Verification items for the finished model (mm, model axes). A direction names the side the tool comes from. Give positions to 0.01 mm unless a question says otherwise; leave off trailing zeros. Write each loop counter-clockwise with the first axis right and the second up, starting at its lowest first coordinate (ties: lowest second). Pieces come first, ordered by that corner, then holes. Notation, with made-up numbers: M 80.5,51 L 107.5,51 A31 ccw 107.5,76 Z; hole C 8,-23.75 d3. An arc over 180 degrees is marked long. Write item = value, one per line.
from build123d import *

# Parameters (mm, degrees)
SKETCH3_R               = 1.7
CUT_EXTRUDE1_DEPTH      = 68.372101051
CIRPATTERN1_COUNT       = 4
BOSS_EXTRUDE1_DEPTH     = 11
SKETCH6_R               = 8.4
CUT_EXTRUDE2_DEPTH      = 3
SKETCH7_W               = 6.9
SKETCH7_H               = 40
CUT_EXTRUDE3_DEPTH      = 4
SKETCH8_R               = 1.7
CUT_EXTRUDE4_DEPTH      = 68.727394753
SKETCH9_R               = 4
BOSS_EXTRUDE2_DEPTH     = 6.5
SKETCH10_R              = 1.7
CUT_EXTRUDE5_DEPTH      = 69.733179761
CUT_EXTRUDE6_DEPTH      = 1
CUT_EXTRUDE6_DEPTH_BACK = 3
SKETCH12_R              = 2.95
CUT_EXTRUDE7_DEPTH      = 3
CIRPATTERN2_COUNT       = 4
CUT_EXTRUDE8_DEPTH      = 3


with BuildPart() as part:
    # Sketch1 → Revolve1 (revolve)
    with BuildSketch(Plane.XY):
        Polygon((25, 0), (47, 0), (47, -5), (35, -5), (35, -11), (25, -11), align=None)
    revolve(axis=Axis((0, -62.255842479, 0), (0, 1, 0)))

    # Sketch3 → Cut-Extrude1 (cut, symmetric)
    with BuildSketch(Plane(origin=(0, 0, 0), x_dir=(1, 0, 0), z_dir=(0, 1, 0))):
        with Locations(Location((21.213203436, 21.213203436, 0), (0, 0, 180))):
            Circle(SKETCH3_R)
    cut_extrude1 = extrude(amount=CUT_EXTRUDE1_DEPTH, both=True, mode=Mode.SUBTRACT)

    # CirPattern1: Cut-Extrude1 ×4 about axis
    cirpattern1_axis = Axis((0, 0, 0), (0, 1, 0))
    for i in range(1, CIRPATTERN1_COUNT):
        add(cut_extrude1.rotate(cirpattern1_axis, i * 360 / CIRPATTERN1_COUNT), mode=Mode.SUBTRACT)

    # Sketch4 → Boss-Extrude1 (add, through all)
    with BuildSketch(Plane(origin=(0, 0, 0), x_dir=(1, 0, 0), z_dir=(0, 1, 0))):
        with BuildLine():
            ThreePointArc((4.118263467, 16.493632287), (-12.020815273, 12.020815288), (-16.493632292, -4.118263447))
            ThreePointArc((-16.493632292, -4.118263447), (-19.405482869, -8.968121999), (-24.255341261, -6.056271155))
            ThreePointArc((-24.255341261, -6.056271155), (17.677669687, -17.677669372), (6.056270723, 24.255341369))
            ThreePointArc((6.056270723, 24.255341369), (8.968122055, 19.405483096), (4.118263467, 16.493632287))
        make_face()
    extrude(amount=-BOSS_EXTRUDE1_DEPTH)

    # Sketch5 → Revolve2 (revolve)
    with BuildSketch(Plane(origin=(0, 0, 0), x_dir=(0, 0, -1), z_dir=(1, 0, 0)), mode=Mode.PRIVATE) as revolve2_sk:
        Polygon((-8.4, 0), (-8.4, 6), (-11.8, 6), (-17, 0), align=None)
    revolve(revolve2_sk.sketch.rotate(Axis((0, 0, 0), (0, -1, 0)), 194.019424572), axis=Axis((0, 0, 0), (0, -1, 0)))

    # Sketch6 → Cut-Extrude2 (cut)
    with BuildSketch(Plane(origin=(0, 0, 0), x_dir=(1, 0, 0), z_dir=(0, 1, 0))):
        with Locations(Location((0, 0, 0), (0, 0, 270))):
            Circle(SKETCH6_R)
    extrude(amount=-CUT_EXTRUDE2_DEPTH, mode=Mode.SUBTRACT)

    # Sketch7 → Cut-Extrude3 (cut)
    with BuildSketch(Plane(origin=(0, 6, 0), x_dir=(1, 0, 0), z_dir=(0, 1, 0))):
        Rectangle(SKETCH7_W, SKETCH7_H)
    extrude(amount=-CUT_EXTRUDE3_DEPTH, mode=Mode.SUBTRACT)

    # Sketch8 → Cut-Extrude4 (cut, through all)
    with BuildSketch(Plane(origin=(0, 2, 0), x_dir=(1, 0, 0), z_dir=(0, 1, 0))):
        with Locations(Location((0, 11, 0), (0, 0, 270))):
            Circle(SKETCH8_R)
        with Locations(Location((0, -11, 0), (0, 0, 270))):
            Circle(SKETCH8_R)
    extrude(amount=-CUT_EXTRUDE4_DEPTH, mode=Mode.SUBTRACT)

    # Sketch9 → Boss-Extrude2 (add)
    with BuildSketch(Plane(origin=(0, 0, 0), x_dir=(1, 0, 0), z_dir=(0, 1, 0))):
        with Locations((43, 0)):
            Circle(SKETCH9_R)
        with Locations(Location((15, 0, 0), (0, 0, 293.578178493))):
            Circle(SKETCH9_R)
    extrude(amount=BOSS_EXTRUDE2_DEPTH)

    # Sketch10 → Cut-Extrude5 (cut, through all)
    with BuildSketch(Plane(origin=(0, 6.5, 0), x_dir=(1, 0, 0), z_dir=(0, 1, 0))):
        with Locations(Location((15, 0, 0), (0, 0, 180))):
            Circle(SKETCH10_R)
        with Locations(Location((43, 0, 0), (0, 0, 180))):
            Circle(SKETCH10_R)
    extrude(amount=-CUT_EXTRUDE5_DEPTH, mode=Mode.SUBTRACT)

    # Sketch11 → Cut-Extrude6 (cut, two sides: drawn at the far end of the back side and taken through both)
    with BuildSketch(Plane(origin=(0, 3.5, 0), x_dir=(1, 0, 0), z_dir=(0, 1, 0)).offset(-CUT_EXTRUDE6_DEPTH_BACK)):
        Polygon((18.35, 0), (16.675, 2.901185103), (13.325, 2.901185103), (11.65, 0), (13.325, -2.901185103), (16.675, -2.901185103), align=None)
        Polygon((41.325, 2.901185103), (44.675, 2.901185103), (46.35, 0), (44.675, -2.901185103), (41.325, -2.901185103), (39.65, 0), align=None)
        Polygon((16.675, -2.901185103), (18.35, 0), (16.675, 2.901185103), (41.325, 2.901185103), (39.65, 0), (41.325, -2.901185103), align=None)
    extrude(amount=CUT_EXTRUDE6_DEPTH + CUT_EXTRUDE6_DEPTH_BACK, mode=Mode.SUBTRACT)

    # Sketch12 → Cut-Extrude7 (cut)
    with BuildSketch(Plane(origin=(0, 0, 0), x_dir=(1, 0, 0), z_dir=(0, 1, 0))):
        with Locations(Location((-21.213203436, 21.213203436, 0), (0, 0, 180))):
            Circle(SKETCH12_R)
    cut_extrude7 = extrude(amount=-CUT_EXTRUDE7_DEPTH, mode=Mode.SUBTRACT)

    # CirPattern2: Cut-Extrude7 ×4 about axis
    cirpattern2_axis = Axis((0, 0, 0), (0, 1, 0))
    for i in range(1, CIRPATTERN2_COUNT):
        add(cut_extrude7.rotate(cirpattern2_axis, i * 360 / CIRPATTERN2_COUNT), mode=Mode.SUBTRACT)

    # Sketch14 → Cut-Extrude8 (cut)
    with BuildSketch(Plane.XZ.offset(11)):
        Polygon((-1.675, 13.901185103), (1.675, 13.901185103), (3.35, 11), (1.675, 8.098814897), (-1.675, 8.098814897), (-3.35, 11), align=None)
        Polygon((-1.675, -8.098814897), (-3.35, -11), (-1.675, -13.901185103), (1.675, -13.901185103), (3.35, -11), (1.675, -8.098814897), align=None)
    extrude(amount=-CUT_EXTRUDE8_DEPTH, mode=Mode.SUBTRACT)


solid = part.part
1) Cross-section at A-A on x = 43. Record the boundary of the cut face in (y, z), plus the area to 3 significant figures.
From the geometry:
outline = M -5,-18.97 L 0,-18.97 L 0,-4 L 6.5,-4 L 6.5,-1.7 L 4.5,-1.7 L 4.5,-2.9 L 0.5,-2.9 L 0.5,-1.7 L -5,-1.7 Z; M -5,1.7 L 0.5,1.7 L 0.5,2.9 L 4.5,2.9 L 4.5,1.7 L 6.5,1.7 L 6.5,4 L 0,4 L 0,18.97 L -5,18.97 Z
area = 193 mm^2
2) Depth check by flat-ended pin: P1, Ø7, axis at x = -21.21, z = -21.21, coming from the +Y side; P2, Ø3.5, axis at x = -21.21, z = 21.21, coming from the +Y side; P3, Ø8, axis at y = 1.5, z = -8.5, coming from the +X side; P4, Ø6, axis at x = -2, z = -21.5, coming from the -Y side. Enter the tip coordinate at first touch or a pass-through.
From the geometry:
P1 = 0
P2 = -3
P3 = 46.76
P4 = through
3) Cross-section at B-B on z = -31. Record the boundary of the cut face in (x, y).
From the geometry:
outline = M -35.33,-5 L -16.25,-5 L -16.25,-11 L 16.25,-11 L 16.25,-5 L 35.33,-5 L 35.33,0 L -35.33,0 Z
4) Cross-section at C-C on x = 26.5. Record the boundary of the cut face in (y, z), plus the area to 3 significant figures.
From the geometry:
outline = M -11,-22.86 L -5,-22.86 L -5,-38.82 L 0,-38.82 L 0,38.82 L -5,38.82 L -5,22.86 L -11,22.86 Z
area = 663 mm^2
5) Cross-section at D-D on z = 38.5. Record the boundary of the cut face in (x, y).
From the geometry:
outline = M -26.96,-5 L 26.96,-5 L 26.96,0 L -26.96,0 Z
6) Draft check along Y on faces 1 (the flat face through (17, 4.5, 0)), 2 (the flat face through (-2.5, -9.52, 9.53)), 3 (the flat face through (-1.4, -8, 12.3)). Enter one of: +Y half, -Y half, draft (parallel to the pull), parting line (faces both ways), or undercut.
From the geometry:
face_1 = undercut
face_2 = draft
face_3 = -Y half
7) Material ranges on probe 1 along X at (y, z) = (-4, -10); probe 2 along X at (y, z) = (-2.5, -11); probe 3 along Z at (x, y) = (-7, -2), recorded low to high. Write a range as from..to.
From the geometry:
probe_1 = -45.92..-22.91, -13.75..-1.37, 1.37..45.92
probe_2 = -45.69..-22.45, -12.96..-1.7, 1.7..45.69
probe_3 = -46.48..-24, -15.49..-4.64, 4.64..46.48
8) Tool access check on faces 4 (the flat face through (42, 2, -2.901)), 5 (the flat face through (-3.45, 4, 11)), 6 (the cylindrical face through (-18.726, -1.479, 22.799)), 7 (the cylindrical face through (-17.42, -5.42, -17.93)), 8 (the flat face through (0, -10, 8.099)). Record the directions out of +Z, -Z, +X, -X, +Y, -Y that give a thin tool (end or side, any length) a straight path to the whole face; none if there is none.
From the geometry:
face_4 = none
face_5 = +Z, -Z, +Y
face_6 = +Y
face_7 = +Y, -Y
face_8 = -Y
